The model under review builds one solid part; all positions refer to its coordinate system, in mm. Round coordinates to 2 decimals unless told otherwise and drop trailing zeros. Order: outer loops, then holes, each group sorted by start corner. A loop starts at its lowest first (then second) coordinate and runs counter-clockwise, first axis right, second up.
```python
from build123d import *

# Parameters (mm, degrees)
SKETCH1_R               = 1
BOSS_EXTRUDE1_DEPTH     = 3
SKETCH2_W               = 50
SKETCH2_H               = 17
CUT_EXTRUDE1_DEPTH      = 178.476759042
SKETCH3_R               = 75
BOSS_EXTRUDE2_DEPTH     = 3
CIRPATTERN1_OUTLINE_R   = 1
CIRPATTERN1_OUTLINE_W   = 17
CIRPATTERN1_OUTLINE_H   = 50
CIRPATTERN1_OUTLINE_W_2 = 50
CIRPATTERN1_OUTLINE_H_2 = 17
CIRPATTERN1_DEPTH       = 3


# Read off the part's stored shape, not the designer's step: CirPattern1
with BuildPart() as part:
    # Sketch1 → Boss-Extrude1 (new body)
    with BuildSketch(Plane(origin=(0, 0, 0), x_dir=(1, 0, 0), z_dir=(0, 1, 0))):
        with BuildLine():
            Line((0, 0), (151.460758228, 13.062875527))
            ThreePointArc((151.460758228, 13.062875527), (167, 30), (151.460758228, 46.937124473))
            Line((151.460758228, 46.937124473), (0, 60))
            Line((0, 60), (0, 0))
        make_face()
        with Locations(Location((140.807611845, 39.192388155, 0), (0, 0, 270))):
            Circle(SKETCH1_R, mode=Mode.SUBTRACT)
        with Locations(Location((140.807611845, 20.807611845, 0), (0, 0, 270))):
            Circle(SKETCH1_R, mode=Mode.SUBTRACT)
        with Locations(Location((159.192388155, 20.807611845, 0), (0, 0, 270))):
            Circle(SKETCH1_R, mode=Mode.SUBTRACT)
        with Locations(Location((159.192388155, 39.192388155, 0), (0, 0, 270))):
            Circle(SKETCH1_R, mode=Mode.SUBTRACT)
    extrude(amount=BOSS_EXTRUDE1_DEPTH)

    # Sketch2 → Cut-Extrude1 (cut, through all)
    with BuildSketch(Plane(origin=(0, 3, 0), x_dir=(1, 0, 0), z_dir=(0, 1, 0))):
        with Locations((65, 30)):
            Rectangle(SKETCH2_W, SKETCH2_H)
    extrude(amount=-CUT_EXTRUDE1_DEPTH, mode=Mode.SUBTRACT)

    # Sketch3 → Boss-Extrude2 (add)
    with BuildSketch(Plane(origin=(0, 3, 0), x_dir=(1, 0, 0), z_dir=(0, 1, 0))):
        with Locations((-58, 30)):
            Circle(SKETCH3_R)
    extrude(amount=-BOSS_EXTRUDE2_DEPTH)

    # CirPattern1 outline → CirPattern1 (add)
    # profile 1 of 3: a face of its own
    with BuildSketch(Plane(origin=(0, 0, 0), x_dir=(1, 0, 0), z_dir=(0, 1, 0))):
        with BuildLine():
            ThreePointArc((-28.961675415, -39.150384708), (-58, -45), (-87.038324585, -39.150384708))
            Line((-87.038324585, -39.150384708), (-74.937124473, -179.460758228))
            ThreePointArc((-74.937124473, -179.460758228), (-58, -195), (-41.062875527, -179.460758228))
            Line((-41.062875527, -179.460758228), (-28.961675415, -39.150384708))
        make_face()
        with Locations((-67.192388155, -187.192388155)):
            Circle(CIRPATTERN1_OUTLINE_R, mode=Mode.SUBTRACT)
        with Locations((-67.192388155, -168.807611845)):
            Circle(CIRPATTERN1_OUTLINE_R, mode=Mode.SUBTRACT)
        with Locations((-48.807611845, -187.192388155)):
            Circle(CIRPATTERN1_OUTLINE_R, mode=Mode.SUBTRACT)
        with Locations((-48.807611845, -168.807611845)):
            Circle(CIRPATTERN1_OUTLINE_R, mode=Mode.SUBTRACT)
        with Locations((-58, -93)):
            Rectangle(CIRPATTERN1_OUTLINE_W, CIRPATTERN1_OUTLINE_H, mode=Mode.SUBTRACT)
    # profile 2 of 3: a face of its own
    with BuildSketch(Plane(origin=(0, 0, 0), x_dir=(1, 0, 0), z_dir=(0, 1, 0))):
        with BuildLine():
            ThreePointArc((-127.150384708, 0.961675415), (-133, 30), (-127.150384708, 59.038324585))
            Line((-127.150384708, 59.038324585), (-267.460758228, 46.937124473))
            ThreePointArc((-267.460758228, 46.937124473), (-283, 30), (-267.460758228, 13.062875527))
            Line((-267.460758228, 13.062875527), (-127.150384708, 0.961675415))
        make_face()
        with Locations((-275.192388155, 20.807611845)):
            Circle(CIRPATTERN1_OUTLINE_R, mode=Mode.SUBTRACT)
        with Locations((-256.807611845, 20.807611845)):
            Circle(CIRPATTERN1_OUTLINE_R, mode=Mode.SUBTRACT)
        with Locations((-275.192388155, 39.192388155)):
            Circle(CIRPATTERN1_OUTLINE_R, mode=Mode.SUBTRACT)
        with Locations((-256.807611845, 39.192388155)):
            Circle(CIRPATTERN1_OUTLINE_R, mode=Mode.SUBTRACT)
        with Locations((-181, 30)):
            Rectangle(CIRPATTERN1_OUTLINE_W_2, CIRPATTERN1_OUTLINE_H_2, mode=Mode.SUBTRACT)
    # profile 3 of 3: a face of its own
    with BuildSketch(Plane(origin=(0, 0, 0), x_dir=(1, 0, 0), z_dir=(0, 1, 0))):
        with BuildLine():
            ThreePointArc((-41.062875527, 239.460758228), (-58, 255), (-74.937124473, 239.460758228))
            Line((-74.937124473, 239.460758228), (-87.038324585, 99.150384708))
            ThreePointArc((-87.038324585, 99.150384708), (-58, 105), (-28.961675415, 99.150384708))
            Line((-28.961675415, 99.150384708), (-41.062875527, 239.460758228))
        make_face()
        with Locations((-58, 153)):
            Rectangle(CIRPATTERN1_OUTLINE_W, CIRPATTERN1_OUTLINE_H, mode=Mode.SUBTRACT)
        with Locations((-67.192388155, 228.807611845)):
            Circle(CIRPATTERN1_OUTLINE_R, mode=Mode.SUBTRACT)
        with Locations((-67.192388155, 247.192388155)):
            Circle(CIRPATTERN1_OUTLINE_R, mode=Mode.SUBTRACT)
        with Locations((-48.807611845, 228.807611845)):
            Circle(CIRPATTERN1_OUTLINE_R, mode=Mode.SUBTRACT)
        with Locations((-48.807611845, 247.192388155)):
            Circle(CIRPATTERN1_OUTLINE_R, mode=Mode.SUBTRACT)
    extrude(amount=CIRPATTERN1_DEPTH)


solid = part.part
```
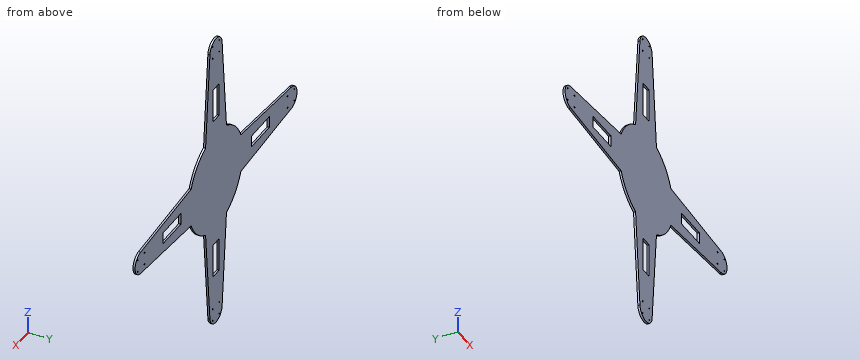
(1) Consider section A-A (z = -157.5). Write out the cut boundary in (x, y), and give its area (3 significant figures).
Data:
outline: (-82.01, 0) - (-66.5, 0) - (-66.5, 3) - (-82.01, 3) - close; (-49.5, 0) - (-33.99, 0) - (-33.99, 3) - (-49.5, 3) - close
area: 93.0 mm2
(2) To check wall thickness, follow probe 1 along X at (y, z) = (2.2, -31.5); probe 2 along X at (y, z) = (2.6, 99); probe 3 along X at (y, z) = (2.6, 67). State the ranges of each line that lie inside material, in increasing order.
Data:
probe 1: x = -282.93 to -206, -156 to 40, 90 to 166.93
probe 2: x = -81.88 to -66.5, -49.5 to -34.12
probe 3: x = -84.64 to -31.36
(3) Consider section D-D (z = 51.5). Write out the cut boundary in (x, y), and give its area (3 significant figures).
Data:
outline: (-85.97, 0) - (-30.03, 0) - (-30.03, 3) - (-85.97, 3) - close
area: 168 mm2
(4) Consider section B-B (y = 1.45). State how many separate pieces and enclosed holes the cut face has, and give its area (3 significant figures).
Data:
separate pieces: 1
enclosed holes: 20
area: 40,700 mm2
(5) Consider section C-C (x = 5). Write out the cut boundary in (y, z), and give its area (3 significant figures).
Data:
outline: (0, -70.69) - (3, -70.69) - (3, 10.69) - (0, 10.69) - close
area: 244 mm2
(6) Insertion check: pin 1 (1.5 mm diameter, centred on y = 1, z = 99, fed in from -X); pin 2 (1.5 mm diameter, centred on x = -56.5, y = 1.5, fed in from +Z); pin 3 (0.9 mm diameter, centred on x = -60, y = 2, fed in from -Z); pin 4 (1.2 mm diameter, centred on x = -48.81, z = 187.19, fed in from -Y). Each pin has a flat end and moves straight along its axis. Give the tip position at first contact, or say it passes through.
Data:
pin 1: stops at x = -81.94
pin 2: stops at z = 194.98
pin 3: stops at z = -254.93
pin 4: passes through
